Design review of the part built by this model. Coordinates are the model's own, in mm. A direction names the side the tool comes from. Coordinates: 2 decimals unless noted, no trailing zeros. Write each loop counter-clockwise with the first axis right and the second up, starting at its lowest first coordinate (ties: lowest second). Pieces come first, ordered by that corner, then holes. Notation, with made-up numbers: M 29,-34 L 69,-34 A7 cw 69,-26 Z; hole C 75,86 d9. An arc over 180 degrees is marked long. One line per question, with ' | ' between items.
from build123d import *

# Parameters (mm, degrees)
P_IDAT_VYSUNUT_M1_DEPTH  = 8
SKICA2_W                 = 1.4
SKICA2_H                 = 2.8
ODEBRAT_VYSUNUT_M1_DEPTH = 4.4
SKICA3_W                 = 2
SKICA3_H                 = 2
P_IDAT_VYSUNUT_M2_DEPTH  = 4
P_IDAT_START             = 8
SKICA5_W                 = 16
SKICA5_H                 = 8
P_IDAT_VYSUNUT_M4_DEPTH  = 16
ODEBRAT_VYSUNUT_M2_DEPTH = 161.57934176
ODEBRAT_VYSUNUT_M3_DEPTH = 161.57934176


with BuildPart() as part:
    # Skica1 → Přidat vysunutím1 (new body)
    with BuildSketch(Plane(origin=(0, 0, 0), x_dir=(1, 0, 0), z_dir=(0, 1, 0))):
        Polygon((0, 0), (0, -55.45), (149.85, -3), (127.147799643, -3), (107, -10.052066008), (107, 0), (92, 0), (92, -15.302316258), (7.3, -44.948729338), (7.3, 0), align=None)
    extrude(amount=P_IDAT_VYSUNUT_M1_DEPTH)

    # Skica2 → Odebrat vysunutím1 (cut)
    with BuildSketch(Plane(origin=(0, 8, 0), x_dir=(1, 0, 0), z_dir=(0, 1, 0))):
        with Locations((0.7, -43)):
            Rectangle(SKICA2_W, SKICA2_H)
    extrude(amount=-ODEBRAT_VYSUNUT_M1_DEPTH, mode=Mode.SUBTRACT)

    # Skica3 → Přidat vysunutím2 (add)
    with BuildSketch(Plane.ZY):
        with Locations((11.4, 4)):
            Rectangle(SKICA3_W, SKICA3_H)
        with Locations((29.2, 4)):
            Rectangle(SKICA3_W, SKICA3_H)
        with Locations((47, 4)):
            Rectangle(SKICA3_W, SKICA3_H)
    extrude(amount=P_IDAT_VYSUNUT_M2_DEPTH)

    # Skica5 → Přidat vysunutím4 (add)
    with BuildSketch(Plane(origin=(0, 8, 0), x_dir=(1, 0, 0), z_dir=(0, 1, 0)).offset(P_IDAT_START)):
        with Locations((8, -7)):
            Rectangle(SKICA5_W, SKICA5_H)
    extrude(amount=-P_IDAT_VYSUNUT_M4_DEPTH)

    # Skica6 → Odebrat vysunutím2 (cut, through all)
    with BuildSketch(Plane.ZY):
        Polygon((3, 16), (11, 16), (11, 8), align=None)
    extrude(amount=-ODEBRAT_VYSUNUT_M2_DEPTH, mode=Mode.SUBTRACT)

    # Skica7 → Odebrat vysunutím3 (cut, through all)
    with BuildSketch(Plane.XZ):
        Polygon((7.3, 11), (16, 11), (16, 3), align=None)
    extrude(amount=-ODEBRAT_VYSUNUT_M3_DEPTH, mode=Mode.SUBTRACT)


solid = part.part
1. Tool access review of faces 5 (the face through (11.711, 6.11, 6.944)), 6 (the face through (92, 4, 8)), 7 (the face through (4, 8, 1)): name each direction out of +Z, -Z, +X, -X, +Y, -Y from which nothing blocks a thin tool from reaching the whole face with its end or side.
Answer sheet:
face 5: +Y, -Y | face 6: -Z, +Y, -Y | face 7: -Z, +X, -X, +Y
2. Insertion check: pin 1 Ø1.6 at (x, z) = (-3, 11.5) entering from +Y; pin 2 Ø0.7 at (x, y) = (0.5, 6.5) entering from +Z; pin 3 Ø2 at (x, y) = (-3, 3.5) entering from +Z. Each pin has a flat end and moves straight along its axis. Give the tip position at first contact, or say it passes through.
Answer sheet:
pin 1: y = 5 | pin 2: z = 55.4 | pin 3: z = 48
3. Take a section at D-D (x = 137.5). Write out the cut boundary in (y, z).
Answer sheet:
outline: M 0,3 L 8,3 L 8,7.32 L 0,7.32 Z
4. Take a section at B-B (z = 19). Write out the cut boundary in (x, y), then the cut area to 3 significant figures.
Answer sheet:
outline: M 0,0 L 7.3,0 L 7.3,8 L 0,8 Z; M 81.44,0 L 104.14,0 L 104.14,8 L 81.44,8 Z | area: 240 mm^2
5. Take a section at A-A (z = 6.5). Write out the cut boundary in (x, y).
Answer sheet:
outline: M 0,0 L 12.19,0 L 12.19,12.5 L 0,12.5 Z; M 92,0 L 107,0 L 107,8 L 92,8 Z; M 117.15,0 L 139.85,0 L 139.85,8 L 117.15,8 Z
6. Draft analysis for pull direction X (two halves, no side actions). For faces 1 (the face through (58, 0, 30)), 2 (the face through (117.21, 3.94, 6.48)), 3 (the face through (10, 10, 3)), 4 (the face through (1.4, 6, 43)), state which applies: pulls with the +X half, pulls with the -X half, needs draft (parallel to the pull), parting line crosses it, or undercut.
Answer sheet:
face 1: needs draft | face 2: undercut | face 3: undercut | face 4: pulls with the -X half
7. Take a section at C-C (y = 11.75). Write out the cut boundary in (x, z), then the cut area to 3 significant figures.
Answer sheet:
outline: M 0,3 L 16,3 L 11.38,7.25 L 0,7.25 Z | area: 58.2 mm^2
8. To check wall thickness, follow line 1 along Y through (x, z) = (96, 10); line 2 along Z through (x, y) = (22, 3.5); line 3 along Z through (x, y) = (52.5, 2.5). State the ranges of each line that lie inside material, in increasing order. Write a range as [from, to].
Answer sheet:
line 1: [0, 8] | line 2: [39.8, 47.75] | line 3: [29.13, 37.07]
